Work out the finished part from the listing and answer in its coordinate system (mm). Coordinates: 2 decimals unless noted, no trailing zeros. Loops run counter-clockwise (first coordinate to the right, second up) from the corner with the lowest first, then second, coordinate; pieces in that order, holes last. Notation, with made-up numbers: (63, 23) -> (118, 23) arc R22 cw to (118, 33) -> close; hole circle Ø5 at (3, 45.5). An arc over 180 degrees is marked (long way). One line per question, with ' | ' between items.
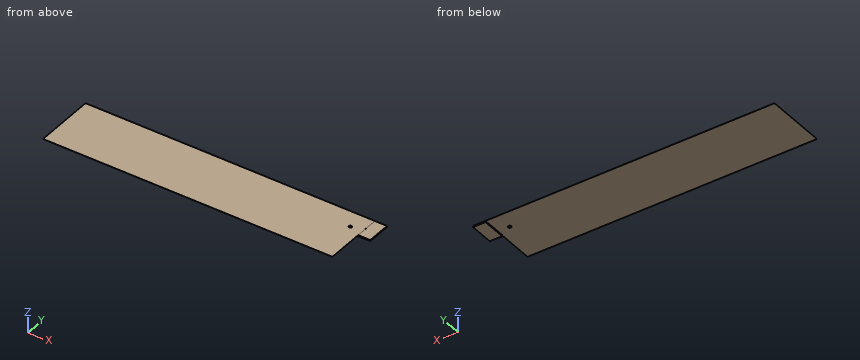
```python
from build123d import *

# Parameters (mm, degrees)
SKETCH1_W           = 609.6
SKETCH1_H           = 128.778
SKETCH1_R           = 0.174798991
SKETCH1_R_2         = 3.175
BOSS_EXTRUDE1_DEPTH = 0.0999998
SKETCH2_W           = 25.4
SKETCH2_H           = 50.8
SKETCH2_W_2         = 0.79375
BOSS_EXTRUDE2_DEPTH = 2.54


with BuildPart() as part:
    # Sketch1 → Boss-Extrude1 (new body)
    with BuildSketch(Plane.XY):
        with Locations((304.8, 64.389)):
            Rectangle(SKETCH1_W, SKETCH1_H)
        with Locations((52.974692136, 90.678)):
            Circle(SKETCH1_R, mode=Mode.SUBTRACT)
        with Locations((584.2, 90.678)):
            Circle(SKETCH1_R_2, mode=Mode.SUBTRACT)
    extrude(amount=BOSS_EXTRUDE1_DEPTH)

    # Sketch2 → Boss-Extrude2 (add)
    with BuildSketch(Plane(origin=(0, 0, 0), x_dir=(-1, 0, 0), z_dir=(0, 0, -1))):
        with Locations((-622.3, 103.378)):
            Rectangle(SKETCH2_W, SKETCH2_H)
        with Locations((-609.203125, 103.378)):
            Rectangle(SKETCH2_W_2, SKETCH2_H)
    extrude(amount=BOSS_EXTRUDE2_DEPTH)


solid = part.part
```
1) Find section A-A (y = 118.5). Write down the section's boundary in (x, z).
Check values:
outline: (0, 0) -> (608.81, 0) -> (608.81, -2.54) -> (635, -2.54) -> (635, 0) -> (609.6, 0) -> (609.6, 0.1) -> (0, 0.1) -> close
2) Flat-ended cylindrical pins translate along their axes: pin 1 (10 mm diameter, centred on x = 584.2, y = 90.678, fed in from -Z); pin 2 (1.3 mm diameter, centred on y = 109.5, z = -2, fed in from -X); pin 3 (20.5 mm diameter, centred on x = 623.5, y = 110, fed in from +Z). Find the tip coordinate at first contact, or state that the pin passes through.
Check values:
pin 1: stops at z = 0 | pin 2: stops at x = 608.81 | pin 3: stops at z = 0
3) Find the intervals of material crossed by line 1 along X through (y, z) = (103.5, -1.85); line 2 along Y through (x, z) = (584.2, 0.05), in increasing order.
Check values:
line 1: x = 608.81 to 635 | line 2: y = 0 to 87.5, 93.85 to 128.78
4) Find section C-C (x = 528). Write down the section's boundary in (y, z), plus the area to 3 significant figures.
Check values:
outline: (0, 0) -> (128.78, 0) -> (128.78, 0.1) -> (0, 0.1) -> close | area: 12.9 mm^2
5) Find section B-B (z = -1.35). Write down the section's boundary in (x, y), plus the area to 3 significant figures.
Check values:
outline: (608.81, 77.98) -> (635, 77.98) -> (635, 128.78) -> (608.81, 128.78) -> close | area: 1,330 mm^2
